Check sheet for the modelled part. Datum: model origin and axes. Units: mm. Face numbers are marked on the shaded views. A direction names the side the tool comes from. Coordinates: 2 decimals unless noted, no trailing zeros. Write each loop counter-clockwise with the first axis right and the second up, starting at its lowest first coordinate (ties: lowest second). Pieces come first, ordered by that corner, then holes. Notation, with made-up numbers: (4, 88.5) -> (56, 88.5) arc R27 ccw to (56, 117.5) -> close; hole circle Ø1 at (-38, -4). An arc over 180 degrees is marked (long way). One line per item, written item: value. Start each with the question number.
1) Scan lines: line 1 along X through (y, z) = (0, -9.5); line 2 along X through (y, z) = (-2.5, 4.5) (3 decimals); line 3 along Y through (x, z) = (63.5, 0). Record each from-to range of solid material in increasing order. Write a range as [from, to].
2) Sectioned sample at D-D on x = 87.5. Enter the section's corners in (y, z), plus the area to 3 significant figures.
3) Sectioned sample at A-A on y = 0. Enter the section's corners in (x, z), plus the area to 3 significant figures.
4) Set-up check for the marked faces 1 and 2: record each of +Z, -Z, +X, -X, +Y, -Y from which the full face is reachable in a straight line by a thin tool's end or side.
5) Gauge pin test, flat ends, axial feed: P1, Ø11, axis at x = 16.67, y = 0, coming from the +Z side; P2, Ø5, axis at y = -15.5, z = -10, coming from the -X side; P3, Ø5, axis at x = 99.5, z = -0.5, coming from the -Y side; P4, Ø1, axis at x = 39.5, y = 3.5, coming from the +Z side. Record the tip position at first contact, or that the pin passes through.
6) Sectioned sample at B-B on z = 0. Enter the section's corners in (x, y), plus the area to 3 significant figures.
7) Sectioned sample at C-C on x = 16. Enter the section's corners in (y, z).
```python
from build123d import *

# Parameters (mm, degrees)
CUT_EXTRUDE1_DEPTH      = 126.099960032
CUT_EXTRUDE1_DEPTH_BACK = 126.099960032
SKETCH3_R               = 6


with BuildPart() as part:
    # Sketch2 → Revolve1 (revolve)
    with BuildSketch(Plane.XY, mode=Mode.PRIVATE) as revolve1_sk:
        Polygon((0, 0), (120, 0), (120, -15), (110, -25), (93.7, -25), (93.7, -18.7), (8.7, -18.7), (0, -10), align=None)
    revolve(revolve1_sk.sketch.rotate(Axis((0, 0, 0), (1, 0, 0)), 270), axis=Axis((0, 0, 0), (1, 0, 0)))

    # Sketch3 → Cut-Extrude1 (cut, two sides: drawn at the far end of the back side and taken through both)
    with BuildSketch(Plane.XY.offset(-CUT_EXTRUDE1_DEPTH_BACK)):
        with Locations((16.669361572, 0)):
            Circle(SKETCH3_R)
    extrude(amount=CUT_EXTRUDE1_DEPTH + CUT_EXTRUDE1_DEPTH_BACK, mode=Mode.SUBTRACT)


solid = part.part
```
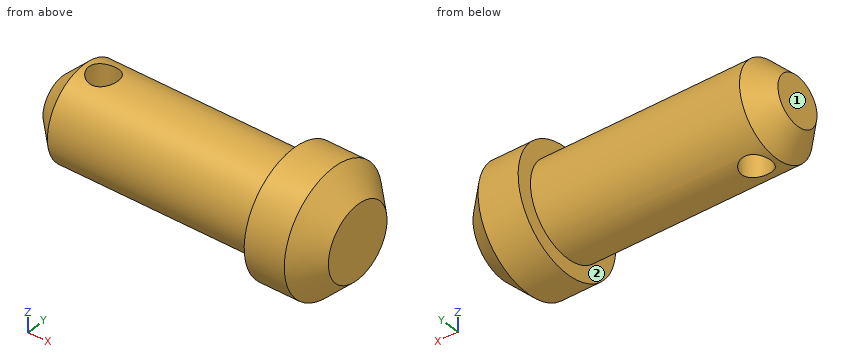
Answers:
1. line 1: x = [0, 10.67], [22.67, 120]
1. line 2: x = [0, 11.215], [22.124, 120]
1. line 3: y = [-18.7, 18.7]
2. outline: circle Ø37.4 at (0, 0)
2. area: 1,100 mm2
3. outline: (0, -10) -> (8.7, -18.7) -> (10.67, -18.7) -> (10.67, 18.7) -> (8.7, 18.7) -> (0, 10) -> close; (22.67, -18.7) -> (93.7, -18.7) -> (93.7, -25) -> (110, -25) -> (120, -15) -> (120, 15) -> (110, 25) -> (93.7, 25) -> (93.7, 18.7) -> (22.67, 18.7) -> close
3. area: 4,190 mm2
4. face 1: +Z, -Z, -X, +Y, -Y
4. face 2: -X
5. P1: passes through
5. P2: stops at x = 5.95
5. P3: stops at y = -25
5. P4: stops at z = 18.46
6. outline: (0, -10) -> (8.7, -18.7) -> (93.7, -18.7) -> (93.7, -25) -> (110, -25) -> (120, -15) -> (120, 15) -> (110, 25) -> (93.7, 25) -> (93.7, 18.7) -> (8.7, 18.7) -> (0, 10) -> close; hole circle Ø12 at (16.67, 0)
6. area: 4,530 mm2
7. outline: (-5.96, -17.72) -> (-5.96, 17.72) arc R18.7 ccw to start; (5.96, -17.72) arc R18.7 ccw to (5.96, 17.72) -> close
